from build123d import *

# Parameters (mm, degrees)
CHAMFER_1_SIZE = 1
CHAMFER_2_SIZE = 1
FILLET_1_R     = 0.2


with BuildPart() as part:
    # 스케치3 → 회전2 (revolve)
    with BuildSketch(Plane(origin=(0, 0, 0), x_dir=(1, 0, 0), z_dir=(0, 1, 0)), mode=Mode.PRIVATE) as revolve_2_sk:
        with BuildLine():
            Line((11.1, 0), (11.1, -2.4))
            Line((11.1, -2.4), (8.6, -2.4))
            Line((8.6, -2.4), (8.6, -4.2))
            Line((8.6, -4.2), (11.1, -6.2))
            Line((11.1, -6.2), (11.1, -8.2))
            Line((11.1, -8.2), (10.075, -8.2))
            Line((10.075, -8.2), (10.075, -13.15))
            Line((10.075, -13.15), (9.575, -13.15))
            ThreePointArc((9.575, -13.15), (8.725, -14), (9.575, -14.85))
            Line((9.575, -14.85), (10.075, -14.85))
            Line((10.075, -14.85), (10.075, -21.8))
            Line((10.075, -21.8), (2.9, -21.8))
            Line((2.9, -21.8), (2.9, -11.8))
            Line((2.9, -11.8), (4.4, -11.8))
            Line((4.4, -11.8), (4.4, -10))
            Line((4.4, -10), (3.4, -10))
            Line((3.4, -10), (3.4, -8.2))
            Line((3.4, -8.2), (5.5, -7.637306696))
            Line((5.5, -7.637306696), (5.5, 0))
            Line((5.5, 0), (11.1, 0))
        make_face()
    revolve(revolve_2_sk.sketch.rotate(Axis((0, 0, 0), (0, 0, 1)), 180), axis=Axis((0, 0, 0), (0, 0, 1)))

    # 모따기1
    chamfer_1_edges = [part.edges().sort_by_distance(p)[0] for p in [
        (10.075, 0, 21.8),
        (5.5, 0, 0),
    ]]
    chamfer(chamfer_1_edges, length=CHAMFER_1_SIZE)

    # 모따기2
    chamfer_2_edges = [part.edges().sort_by_distance(p)[0] for p in [
        (11.1, 0, 0),
    ]]
    chamfer(chamfer_2_edges, length=CHAMFER_2_SIZE)

    # 필렛1
    fillet_1_edges = [part.edges().sort_by_distance(p)[0] for p in [
        (11.1, 0, 2.4),
    ]]
    fillet(fillet_1_edges, radius=FILLET_1_R)


solid = part.part
The listing builds one solid part. Answer for the finished solid, in the listing's coordinates (mm). A direction names the side the tool comes from. Round coordinates to 2 decimals unless told otherwise and drop trailing zeros. Write each loop counter-clockwise with the first axis right and the second up, starting at its lowest first coordinate (ties: lowest second). Pieces come first, ordered by that corner, then holes. Notation, with made-up numbers: (7, 36.25) - (18, 36.25) arc R9 cw to (18, 40.25) - close; hole circle Ø8 at (-32.75, 68.25). An arc over 180 degrees is marked (long way). Use a Markdown table: item, result. Add a question column.
1. Flat-ended cylindrical pins translate along their axes: P1, Ø9, axis at x = 0, y = 0, coming from the -Z side; P2, Ø1.5, axis at x = -5, z = 4, coming from the +Y side; P3, Ø6.5, axis at x = 0, y = 0, coming from the -Z side; P4, Ø7, axis at x = 0, y = 0, coming from the +Z side. Find the tip coordinate at first contact, or state that the pin passes through.
2. For a pull along X with two mould halves and no side action, classify faces 6 (the face through (-2.766, -0.871, 16.73)), 7 (the face through (1.14, -8.682, 4.325)), 8 (the face through (-9, 4, 13.15)) as +X half, -X half, draft (parallel to the pull), parting line (faces both ways), or undercut.
3. Consider line 1 (Y direction, x = 0, z = 18.75) (3 decimals); line 2 (Z direction, x = -8.25, y = -4.5); line 3 (Z direction, x = -7.25, y = -6.25). Determine where each line is inside the solid, lowest interval first.
4. The part is cut by section A-A (z = 16.5). Write down the section's boundary in (x, y) (3 decimals), and give its area (3 significant figures).
5. A tool of negligible diameter and unlimited length cuts with its end or side. For faces 1 (the face through (3, 10, 8.2)), 2 (the face through (-2, 3, 10)), 3 (the face through (-4, 0, 21.8)), 4 (the face through (1.445, -11.006, 7.214)), 5 (the face through (0.74, 3.32, 9.09)), from which of +Z, -Z, +X, -X, +Y, -Y can it reach the whole face along a straight path? Write none if from no direction.
Reported:
| question | item | result |
|---|---|---|
| 1 | P1 | z = 7.91 |
| 1 | P2 | y = 7.92 |
| 1 | P3 | z = 11.8 |
| 1 | P4 | z = 21.8 |
| 2 | face 6 | undercut |
| 2 | face 7 | parting line |
| 2 | face 8 | draft |
| 3 | line 1 | -10.075 to -2.9, 2.9 to 10.075 |
| 3 | line 2 | 0 to 2.4, 4.84 to 13.17, 14.83 to 21.48 |
| 3 | line 3 | 0 to 2.4, 4.98 to 13.15, 14.85 to 21.3 |
| 4 | outline | circle Ø20.15 at (0, 0); hole circle Ø5.8 at (0, 0) |
| 4 | area | 292 mm^2 |
| 5 | face 1 | +Z |
| 5 | face 2 | none |
| 5 | face 3 | +Z, +X, -X, +Y, -Y |
| 5 | face 4 | +Z, -Z |
| 5 | face 5 | -Z |
